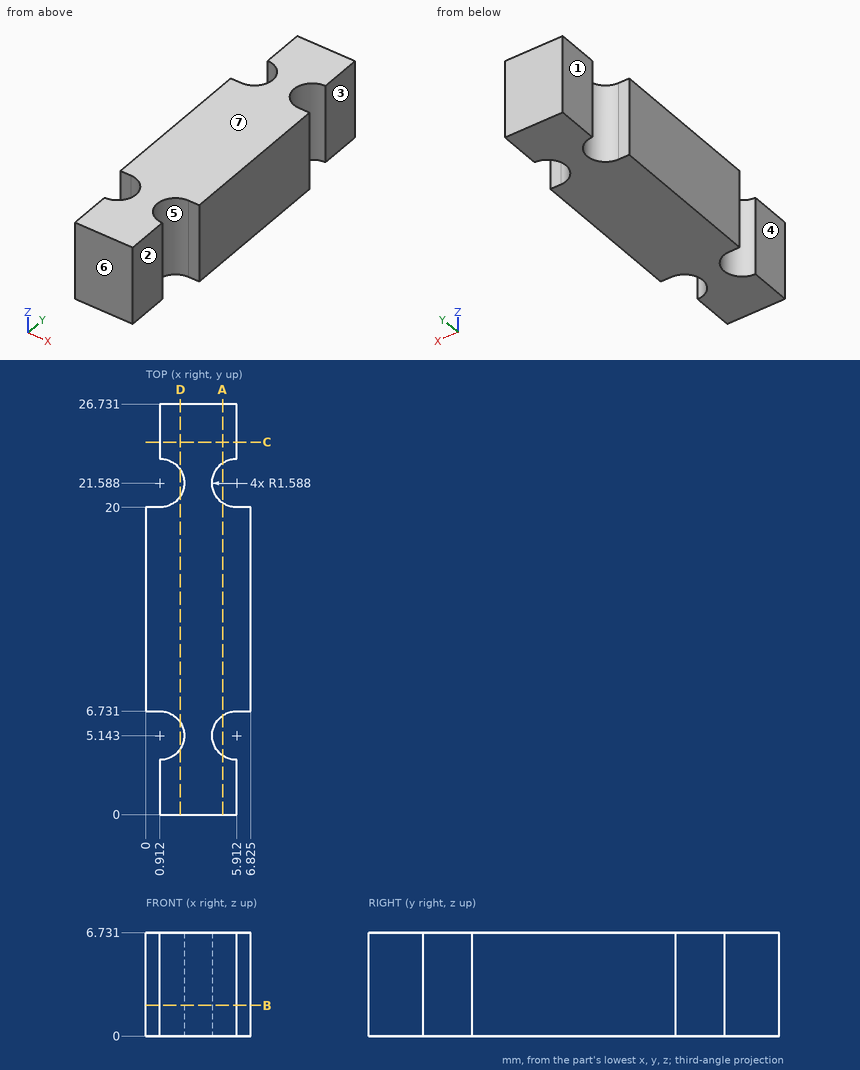
The figure shows three views and two pictorial views of one solid part (mm, origin at its lowest corner). Answer the questions. A direction names the side the tool comes from. Round coordinates to 2 decimals unless told otherwise and drop trailing zeros. Write each loop counter-clockwise with the first axis right and the second up, starting at its lowest first coordinate (ties: lowest second). Pieces come first, ordered by that corner, then holes. Notation, with made-up numbers: (59, 68) - (80, 68) arc R23 ccw to (80, 93) - close; hole circle Ø3 at (16.5, -14.5). An arc over 180 degrees is marked (long way). One line per question, with ' | ' between items. Start each with the question number.
1. For the marked faces 1, 2, 3 and 4, determine the directions among +Z, -Z, +X, -X, +Y, -Y from which every point of the face is accessible in a straight line to the end or side of a thin tool.
2. Section C-C (y = 24.25) is taken. Determine the outline of the cut face in (x, z).
3. Section A-A (x = 5) is taken. Determine the outline of the cut face in (y, z), and give its area (3 significant figures).
4. Each of these flat-tipped pins is pushed along its axis until it touches: pin 1 (1.8 mm diameter, centred on y = 25, z = 2, fed in from +X); pin 2 (4 mm diameter, centred on y = 24.5, z = 3, fed in from -X); pin 3 (1 mm diameter, centred on x = 6.5, z = 2, fed in from +Y). Where does it stop, or does it pass through?
5. For a pull along Y with two mould halves and no side action, classify the marked faces 5, 6 and 7 as +Y half, -Y half, draft (parallel to the pull), parting line (faces both ways), or undercut.
6. Find the intervals of material crossed by probe 1 along Y at (x, z) = (5.25, 2) (1 decimal); probe 2 along Y at (x, z) = (2, 3) (1 decimal); probe 3 along X at (y, z) = (5.25, 2.5), in increasing order. Write a range as [from, to].
7. Section B-B (z = 2) is taken. Determine the outline of the cut face in (x, y) (1 decimal), and give its area (3 significant figures).
8. Section D-D (x = 2.25) is taken. Determine the outline of the cut face in (y, z) (1 decimal), and give its area (3 significant figures).
Filled in:
1) face 1: +Z, -Z, -X, +Y | face 2: +Z, -Z, +X, -Y | face 3: +Z, -Z, +X, +Y | face 4: +Z, -Z, -X, -Y
2) outline: (0.91, 0) - (5.91, 0) - (5.91, 6.73) - (0.91, 6.73) - close
3) outline: (0, 0) - (3.84, 0) - (3.84, 6.73) - (0, 6.73) - close; (6.44, 0) - (20.29, 0) - (20.29, 6.73) - (6.44, 6.73) - close; (22.89, 0) - (26.73, 0) - (26.73, 6.73) - (22.89, 6.73) - close | area: 145 mm²
4) pin 1: x = 5.91 | pin 2: x = 0.91 | pin 3: y = 20
5) face 5: undercut | face 6: -Y half | face 7: draft
6) probe 1: [0, 3.7], [6.6, 20.1], [23, 26.7] | probe 2: [0, 4], [6.3, 20.4], [22.7, 26.7] | probe 3: [2.5, 4.33]
7) outline: (0, 6.7) - (0.9, 6.7) arc R1.6 cw to (0.9, 3.6) - (0.9, 0) - (5.9, 0) - (5.9, 3.6) arc R1.6 cw to (5.9, 6.7) - (6.8, 6.7) - (6.8, 20) - (5.9, 20) arc R1.6 cw to (5.9, 23.2) - (5.9, 26.7) - (0.9, 26.7) - (0.9, 23.2) arc R1.6 cw to (0.9, 20) - (0, 20) - close | area: 142 mm²
8) outline: (0, 0) - (4.3, 0) - (4.3, 6.7) - (0, 6.7) - close; (6, 0) - (20.7, 0) - (20.7, 6.7) - (6, 6.7) - close; (22.4, 0) - (26.7, 0) - (26.7, 6.7) - (22.4, 6.7) - close | area: 157 mm²
